Could you check a few things on this model? Use its own coordinates, in mm. A direction names the side the tool comes from. Give positions to 0.01 mm unless a question says otherwise; leave off trailing zeros. Order: outer loops, then holes, each group sorted by start corner. A loop starts at its lowest first (then second) coordinate and runs counter-clockwise, first axis right, second up.
(1) On a 3-axis mill with a long thin cutter (end or side, diameter ignored), from which of +Z, -Z, +X, -X, +Y, -Y can I reach the whole of each face in a straight line? I mean faces 1 (the cylindrical face through (27.699, 23.768, 2.785)), 2 (the flat face through (14, 1, 40)). Say none if no direction works.
(2) Imagine slicing it at A-A, the plane x = 17. Write out the boundary of the cut face in (y, z), then the cut area to 3 significant figures.
(3) Imagine slicing it at B-B, the plane y = 25. Write out the boundary of the cut face in (x, z), then the cut area to 3 significant figures.
(4) If I drill on probe 1 along X at (y, z) = (1.7, 20); probe 2 along Z at (x, y) = (4, 1.4); probe 3 along X at (y, z) = (14.5, 5), over which ranges is the centre line in solid material (lowest first)?
(5) If we mould it in two halves opening along Z, with no side actions, what happens to faces 3 (the cylindrical face through (12.89, 1.27, 28.99)), 4 (the flat face through (28, 13, 13)), 5 (the cylindrical face through (4.806, 1.267, 28.735)), 6 (the flat face through (29.11, 19.76, 21.51))? For each: released by +Z, released by -Z, zero draft, split by the parting line, or undercut.
(6) Will these pins go through, and if not, where does the flat tip stop? pin 1 (8 mm diameter, centred on x = 4.5, y = 4, fed in from +Z); pin 2 (2.5 mm diameter, centred on x = 4, z = 20, fed in from -Y); pin 3 (13 mm diameter, centred on x = 18.5, z = 20.5, fed in from +Y); pin 4 (1.5 mm diameter, centred on x = 10, y = 15, fed in from +Z).
(7) Imagine slicing it at C-C, the plane z = 30. Write out the boundary of the cut face in (x, y), then the cut area to 3 significant figures.
(8) Imagine slicing it at D-D, the plane z = 17.5. Write out the boundary of the cut face in (x, y).
from build123d import *

# Parameters (mm, degrees)
BOSS_EXTRUDE1_DEPTH            = 28
BOSS_EXTRUDE2_DEPTH            = 2.5
BOSS_EXTRUDE3_DEPTH            = 2.5
SKETCH4_W                      = 33
SKETCH4_H                      = 40
BOSS_EXTRUDE4_DEPTH            = 2.5
F_3_0_3_DIAMETER_HOLE1_D       = 3
F_3_0_3_DIAMETER_HOLE1_DEPTH   = 37.500025
F_7_5_7_5_DIAMETER_HOLE1_D     = 7.5
F_7_5_7_5_DIAMETER_HOLE1_DEPTH = 40
F_3_0_3_DIAMETER_HOLE2_D       = 3
F_3_0_3_DIAMETER_HOLE2_DEPTH   = 40
FILLET1_R                      = 1


with BuildPart() as part:
    # Boss-Extrude1: read off the stored shape, not the designer's step
    # Boss-Extrude1 outline → Boss-Extrude1 (new body)
    with BuildSketch(Plane.YZ):
        Polygon((2.5, 0), (37.5, 0), (37.5, 2.5), (10, 2.5), (2.5, 10), align=None)
    extrude(amount=BOSS_EXTRUDE1_DEPTH)

    # Sketch2 → Boss-Extrude2 (add)
    with BuildSketch(Plane(origin=(28, 0, 0), x_dir=(0, 0, -1), z_dir=(1, 0, 0))):
        Polygon((0, 2.5), (-40, 2.5), (-2.5, 37.5), (0, 37.5), align=None)
    extrude(amount=BOSS_EXTRUDE2_DEPTH)

    # Sketch3 → Boss-Extrude3 (add)
    with BuildSketch(Plane.ZY):
        Polygon((40, 2.5), (0, 2.5), (0, 37.5), (2.5, 37.5), align=None)
    extrude(amount=BOSS_EXTRUDE3_DEPTH)

    # Sketch4 → Boss-Extrude4 (add)
    with BuildSketch(Plane.XZ.offset(-2.5)):
        with Locations((14, 20)):
            Rectangle(SKETCH4_W, SKETCH4_H)
    extrude(amount=BOSS_EXTRUDE4_DEPTH)

    # Ø3.0 (3) Diameter Hole1
    with Locations(Plane(origin=(0, 0, 0), x_dir=(-1, 0, 0), z_dir=(0, -1, 0))):
        with Locations((-4, -30), (-4, -20), (-14, -30), (-14, -20), (-24, -30), (-24, -20)):
            Hole(F_3_0_3_DIAMETER_HOLE1_D / 2, depth=F_3_0_3_DIAMETER_HOLE1_DEPTH)

    # Ø7.5 (7.5) Diameter Hole1
    with Locations(Plane(origin=(0, 0, 0), x_dir=(-1, 0, 0), z_dir=(0, 0, -1))):
        with Locations((-14, 25)):
            Hole(F_7_5_7_5_DIAMETER_HOLE1_D / 2, depth=F_7_5_7_5_DIAMETER_HOLE1_DEPTH)

    # Ø3.0 (3) Diameter Hole2
    with Locations(Plane(origin=(0, 0, 0), x_dir=(-1, 0, 0), z_dir=(0, 0, -1))):
        with Locations((-22.5, 25), (-5.5, 25)):
            Hole(F_3_0_3_DIAMETER_HOLE2_D / 2, depth=F_3_0_3_DIAMETER_HOLE2_DEPTH)

    # Fillet1
    fillet1_edges = [part.edges().sort_by_distance(p)[0] for p in [
        (14, 2.5, 10),
        (0, 6.25, 6.25),
        (28, 6.25, 6.25),
        (14, 10, 2.5),
        (0, 23.75, 2.5),
        (28, 23.75, 2.5),
        (28, 2.5, 25),
        (0, 2.5, 25),
    ]]
    fillet(fillet1_edges, radius=FILLET1_R)


solid = part.part
Answer block:
1. face 1: +Z, +Y
1. face 2: +Z, +X, -X, +Y, -Y
2. outline: (0, 0) - (22.75, 0) - (22.75, 2.5) - (10.41, 2.5) arc R1 cw to (9.71, 2.79) - (2.79, 9.71) arc R1 cw to (2.5, 10.41) - (2.5, 40) - (0, 40) - close; (27.25, 0) - (37.5, 0) - (37.5, 2.5) - (27.25, 2.5) - close
2. area: 204 mm2
3. outline: (-2.5, 0) - (4, 0) - (4, 2.5) - (1, 2.5) arc R1 cw to (0, 3.5) - (0, 15.89) - (-2.5, 15.89) - close; (7, 0) - (10.25, 0) - (10.25, 2.5) - (7, 2.5) - close; (17.75, 0) - (21, 0) - (21, 2.5) - (17.75, 2.5) - close; (24, 0) - (30.5, 0) - (30.5, 15.89) - (28, 15.89) - (28, 3.5) arc R1 cw to (27, 2.5) - (24, 2.5) - close
3. area: 116 mm2
4. probe 1: x = -2.5 to 2.5, 5.5 to 12.5, 15.5 to 22.5, 25.5 to 30.5
4. probe 2: z = 0 to 18.5, 21.5 to 28.5, 31.5 to 40
4. probe 3: x = -2.5 to 0, 28 to 30.5
5. face 3: undercut
5. face 4: zero draft
5. face 5: undercut
5. face 6: released by +Z
6. pin 1: stops at z = 40
6. pin 2: passes through
6. pin 3: stops at y = 2.5
6. pin 4: stops at z = 2.5
7. outline: (-2.5, 0) - (2.5, 0) - (2.5, 2.5) - (1, 2.5) arc R1 cw to (0, 3.5) - (0, 11.83) - (-2.5, 11.83) - close; (5.5, 0) - (12.5, 0) - (12.5, 2.5) - (5.5, 2.5) - close; (15.5, 0) - (22.5, 0) - (22.5, 2.5) - (15.5, 2.5) - close; (25.5, 0) - (30.5, 0) - (30.5, 11.83) - (28, 11.83) - (28, 3.5) arc R1 cw to (27, 2.5) - (25.5, 2.5) - close
7. area: 107 mm2
8. outline: (-2.5, 0) - (30.5, 0) - (30.5, 23.5) - (28, 23.5) - (28, 3.5) arc R1 cw to (27, 2.5) - (1, 2.5) arc R1 cw to (0, 3.5) - (0, 23.5) - (-2.5, 23.5) - close
